from build123d import *

# Parameters (mm, degrees)
ESQUISSE1_W        = 2
ESQUISSE1_H        = 6
ESQUISSE1_W_2      = 15
ESQUISSE1_W_3      = 8
BOSS_EXTRU_2_DEPTH = 2
ESQUISSE1_4_W      = 2
ESQUISSE1_4_H      = 6
BOSS_EXTRU_3_DEPTH = 15
ESQUISSE1_5_W      = 2
ESQUISSE1_5_H      = 6
BOSS_EXTRU_4_DEPTH = 15


with BuildPart() as part:
    # Esquisse1 → Boss.-Extru.2 (new body)
    with BuildSketch(Plane(origin=(0, 0, 0), x_dir=(0, 0, -1), z_dir=(1, 0, 0))):
        with Locations((-18.778399311, -28.757343568)):
            Rectangle(ESQUISSE1_W, ESQUISSE1_H)
        with Locations((-10.278399311, -28.757343568)):
            Rectangle(ESQUISSE1_W_2, ESQUISSE1_H)
        with Locations((-23.778399311, -28.757343568)):
            Rectangle(ESQUISSE1_W_3, ESQUISSE1_H)
    extrude(amount=BOSS_EXTRU_2_DEPTH)

    # Esquisse1_4 → Boss.-Extru.3 (add)
    with BuildSketch(Plane(origin=(0, 0, 0), x_dir=(0, 0, -1), z_dir=(1, 0, 0))):
        with Locations((-28.778399311, -28.757343568)):
            Rectangle(ESQUISSE1_4_W, ESQUISSE1_4_H)
    extrude(amount=BOSS_EXTRU_3_DEPTH)

    # Esquisse1_5 → Boss.-Extru.4 (add)
    with BuildSketch(Plane(origin=(0, 0, 0), x_dir=(0, 0, -1), z_dir=(1, 0, 0))):
        with Locations((-18.778399311, -28.757343568)):
            Rectangle(ESQUISSE1_5_W, ESQUISSE1_5_H)
    extrude(amount=-BOSS_EXTRU_4_DEPTH)


solid = part.part
Geometry: final body of the model. Coordinates: model frame, mm. A direction names the side the tool comes from. Give positions to 0.01 mm unless a question says otherwise; leave off trailing zeros. Write each loop counter-clockwise with the first axis right and the second up, starting at its lowest first coordinate (ties: lowest second). Pieces come first, ordered by that corner, then holes. Notation, with made-up numbers: M 25.5,11.25 L 64.5,11.25 A23 cw 64.5,30.25 Z; hole C 57,-12 d9. An arc over 180 degrees is marked long. Answer in a Markdown table with one row per item. Add a question column.
(1) Section C-C on z = 28.25. Return loops of the section in (x, y), and give its area (3 significant figures).
(2) Section B-B on x = -4.5. Return loops of the section in (y, z).
(3) Reachability of faces 1 (the flat face through (0, -29, 10)), 2 (the flat face through (-15, -29, 19)), 3 (the flat face through (2, -29, 15)), 4 (the flat face through (1, -29, 2.778)), 5 (the flat face through (0, -29, 25)) from +Z, -Z, +X, -X, +Y, -Y: full face, straight path, thin tool, end or side. Return the list, or none.
(4) Ray query, line 1 (Z direction, x = 6.5, y = -28.3); line 2 (X direction, y = -30.9, z = 24); line 3 (Z direction, x = -11.75, y = -31). Return the intervals inside material, ascending.
(5) Section A-A on y = -30.45. Return loops of the section in (x, z), and give its area (3 significant figures).
(6) First-contact query: pin 1 (8 mm diameter, centred on x = -10, z = 14, fed in from -Y); pin 2 (3 mm diameter, centred on x = 9, y = -29, fed in from -Z). Flat tips, straight axial feed; report the tip coordinate or a pass-through.
Result set:
| question | item | result |
|---|---|---|
| 1 | outline | M 0,-31.76 L 15,-31.76 L 15,-25.76 L 0,-25.76 Z |
| 1 | area | 90.0 mm^2 |
| 2 | outline | M -31.76,17.78 L -25.76,17.78 L -25.76,19.78 L -31.76,19.78 Z |
| 3 | face 1 | -Z, -X, +Y, -Y |
| 3 | face 2 | +Z, -Z, -X, +Y, -Y |
| 3 | face 3 | -Z, +X, +Y, -Y |
| 3 | face 4 | -Z, +X, -X, +Y, -Y |
| 3 | face 5 | +Z, -X, +Y, -Y |
| 4 | line 1 | z = 27.78 to 29.78 |
| 4 | line 2 | x = 0 to 2 |
| 4 | line 3 | z = 17.78 to 19.78 |
| 5 | outline | M -15,17.78 L 0,17.78 L 0,2.78 L 2,2.78 L 2,27.78 L 15,27.78 L 15,29.78 L 0,29.78 L 0,19.78 L -15,19.78 Z |
| 5 | area | 110 mm^2 |
| 6 | pin 1 | stops at y = -31.76 |
| 6 | pin 2 | stops at z = 27.78 |
